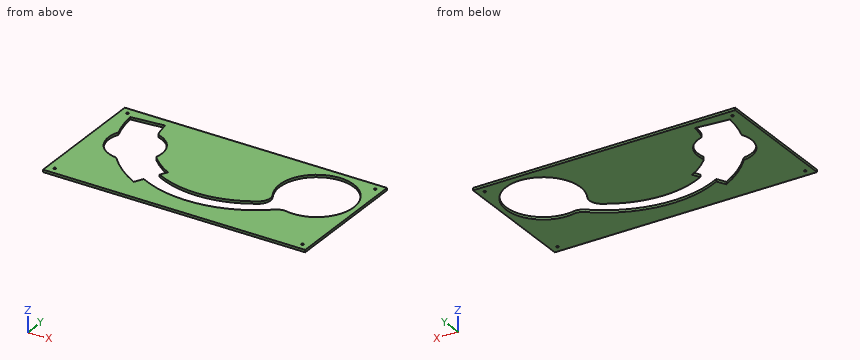
from build123d import *

# Parameters (mm, degrees)
F0_W     = 550
F0_H     = 270
F1_DEPTH = 5
F3_DEPTH = 25
F4_R     = 25
F2_R     = 2.5
F5_DEPTH = 25
F6_R     = 5


with BuildPart() as f1:
    # F0 (on Top) → F1 (new body)
    with BuildSketch(Plane.XY):
        with Locations((275, -135)):
            Rectangle(F0_W, F0_H)
    extrude(amount=-F1_DEPTH)

    # F2 (on face) → F3 (cut)
    with BuildSketch(Plane.XY):
        with BuildLine():
            ThreePointArc((445.5878496959, -168.1072144083), (452.1119253863, -169.1179747106), (458.6981361528, -169.5729777234))
            ThreePointArc((458.6981361528, -169.5729777234), (515.1450884683, -147.5010120731), (538.711061865, -91.6612861494))
            ThreePointArc((538.711061865, -91.6612861494), (531.7751165183, -59.5200686387), (512.2017629268, -33.0994511193))
            ThreePointArc((512.2017629268, -33.0994511193), (489.778644371, -105.9735057557), (445.5878496959, -168.1072144083))
        make_face()
        with BuildLine():
            ThreePointArc((434.4818086721, -165.032732216), (439.9779290015, -166.7755154888), (445.5878496959, -168.1072144083))
            ThreePointArc((445.5878496959, -168.1072144083), (489.778644371, -105.9735057557), (512.2017629268, -33.0994511193))
            ThreePointArc((512.2017629268, -33.0994511193), (507.7316897495, -29.4576002162), (503.004614878, -26.1561769822))
            ThreePointArc((503.004614878, -26.1561769822), (480.8108512866, -101.5487247221), (434.4818086721, -165.032732216))
        make_face()
        with BuildLine():
            ThreePointArc((406.011915497, -147.1219833941), (419.2691571527, -157.6314611673), (434.4818086721, -165.032732216))
            ThreePointArc((434.4818086721, -165.032732216), (480.8108512866, -101.5487247221), (503.004614878, -26.1561769822))
            ThreePointArc((503.004614878, -26.1561769822), (487.87511248, -18.5863859301), (471.4686275556, -14.459543092))
            ThreePointArc((471.4686275556, -14.459543092), (451.6655237624, -87.1681863628), (406.011915497, -147.1219833941))
        make_face()
        with BuildLine():
            ThreePointArc((396.3969974723, -135.5978207964), (400.9264158373, -141.5918788666), (406.011915497, -147.1219833941))
            ThreePointArc((406.011915497, -147.1219833941), (451.6655237624, -87.1681863628), (471.4686275556, -14.459543092))
            ThreePointArc((471.4686275556, -14.459543092), (463.9857274878, -13.7882983897), (456.4729635167, -13.8406471114))
            ThreePointArc((456.4729635167, -13.8406471114), (438.2138341358, -80.5310148123), (396.3969974723, -135.5978207964))
        make_face()
        with BuildLine():
            ThreePointArc((395.2793152892, -133.9137271289), (395.8326968589, -134.7593972826), (396.3969974723, -135.5978207964))
            ThreePointArc((396.3969974723, -135.5978207964), (438.2138341358, -80.5310148123), (456.4729635167, -13.8406471114))
            ThreePointArc((456.4729635167, -13.8406471114), (391.3304963156, -56.2714595868), (395.2793152892, -133.9137271289))
        make_face()
        with BuildLine():
            ThreePointArc((26.1547087534, -24.0004380043), (30.8880481953, -53.9384370008), (39.2095922874, -83.0835942334))
            ThreePointArc((39.2095922874, -83.0835942334), (42.4819606163, -77.1205988593), (46.4524007703, -71.5977994519))
            ThreePointArc((46.4524007703, -71.5977994519), (40.2678425285, -47.5506492992), (36.6062109858, -22.9924196081))
            Line((36.6062109858, -22.9924196081), (26.1547087534, -24.0004380043))
        make_face()
        with BuildLine():
            ThreePointArc((36.6062109858, -22.9924196081), (40.2678425285, -47.5506492992), (46.4524007703, -71.5977994519))
            ThreePointArc((46.4524007703, -71.5977994519), (50.2625511055, -67.3805241048), (54.4801240278, -63.5707031676))
            ThreePointArc((54.4801240278, -63.5707031676), (49.5613274278, -42.9843565598), (46.5600226356, -22.0324020879))
            Line((46.5600226356, -22.0324020879), (36.6062109858, -22.9924196081))
        make_face()
        with BuildLine():
            ThreePointArc((46.5600226356, -22.0324020879), (49.5613274278, -42.9843565598), (54.4801240278, -63.5707031676))
            ThreePointArc((54.4801240278, -63.5707031676), (68.7018719367, -55.1253458568), (84.76908962, -51.1976633843))
            ThreePointArc((84.76908962, -51.1976633843), (81.1661428415, -35.1772059589), (78.9099104977, -18.9123451474))
            Line((78.9099104977, -18.9123451474), (46.5600226356, -22.0324020879))
        make_face()
        with BuildLine():
            ThreePointArc((78.9099104977, -18.9123451474), (81.1661428415, -35.1772059589), (84.76908962, -51.1976633843))
            ThreePointArc((84.76908962, -51.1976633843), (92.7043581114, -51.0322504264), (100.5834584289, -51.9891337337))
            ThreePointArc((100.5834584289, -51.9891337337), (96.3763447636, -34.89397928), (93.8406279725, -17.4723188671))
            Line((93.8406279725, -17.4723188671), (78.9099104977, -18.9123451474))
        make_face()
        with BuildLine():
            ThreePointArc((93.8406279725, -17.4723188671), (96.3763447636, -34.89397928), (100.5834584289, -51.9891337337))
            ThreePointArc((100.5834584289, -51.9891337337), (101.702824577, -52.2182469254), (102.8172889589, -52.4701250099))
            ThreePointArc((102.8172889589, -52.4701250099), (98.4454239564, -35.0497029669), (95.8313903025, -17.2803153631))
            Line((95.8313903025, -17.2803153631), (93.8406279725, -17.4723188671))
        make_face()
        with BuildLine():
            ThreePointArc((102.8172889589, -52.4701250099), (119.1726628165, -90.0990620723), (143.6244940218, -123.0466433063))
            ThreePointArc((143.6244940218, -123.0466433063), (145.375436454, -115.11981647), (145.9631920321, -107.023216784))
            ThreePointArc((145.9631920321, -107.023216784), (133.8730301026, -72.2467564476), (102.8172889589, -52.4701250099))
        make_face()
        with BuildLine():
            ThreePointArc((100.5834584289, -51.9891337337), (117.4412479589, -91.100162762), (142.9268949098, -125.2225814773))
            ThreePointArc((142.9268949098, -125.2225814773), (143.2867819227, -124.1381669965), (143.6244940218, -123.0466433063))
            ThreePointArc((143.6244940218, -123.0466433063), (119.1726628165, -90.0990620723), (102.8172889589, -52.4701250099))
            ThreePointArc((102.8172889589, -52.4701250099), (101.702824577, -52.2182469254), (100.5834584289, -51.9891337337))
        make_face()
        with BuildLine():
            ThreePointArc((84.76908962, -51.1976633843), (104.455636527, -98.6084179347), (135.7230627314, -139.3231306894))
            ThreePointArc((135.7230627314, -139.3231306894), (139.8253147464, -132.5284727964), (142.9268949098, -125.2225814773))
            ThreePointArc((142.9268949098, -125.2225814773), (117.4412479589, -91.100162762), (100.5834584289, -51.9891337337))
            ThreePointArc((100.5834584289, -51.9891337337), (92.7043581114, -51.0322504264), (84.76908962, -51.1976633843))
        make_face()
        with BuildLine():
            ThreePointArc((54.4801240278, -63.5707031676), (76.3201450911, -114.8763041421), (109.8887146149, -159.4004812994))
            ThreePointArc((109.8887146149, -159.4004812994), (124.3031821577, -151.2884347545), (135.7230627314, -139.3231306894))
            ThreePointArc((135.7230627314, -139.3231306894), (104.455636527, -98.6084179347), (84.76908962, -51.1976633843))
            ThreePointArc((84.76908962, -51.1976633843), (68.7018719367, -55.1253458568), (54.4801240278, -63.5707031676))
        make_face()
        with BuildLine():
            ThreePointArc((46.4524007703, -71.5977994519), (67.6630708031, -119.8818075906), (98.9269281749, -162.353082441))
            ThreePointArc((98.9269281749, -162.353082441), (104.4827523758, -161.1549696004), (109.8887146149, -159.4004812994))
            ThreePointArc((109.8887146149, -159.4004812994), (76.3201450911, -114.8763041421), (54.4801240278, -63.5707031676))
            ThreePointArc((54.4801240278, -63.5707031676), (50.2625511055, -67.3805241048), (46.4524007703, -71.5977994519))
        make_face()
        with BuildLine():
            ThreePointArc((39.2095922874, -83.0835942334), (58.5731428007, -125.1375862115), (85.359218008, -162.8998889056))
            ThreePointArc((85.359218008, -162.8998889056), (92.159689712, -163.0387878421), (98.9269281749, -162.353082441))
            ThreePointArc((98.9269281749, -162.353082441), (67.6630708031, -119.8818075906), (46.4524007703, -71.5977994519))
            ThreePointArc((46.4524007703, -71.5977994519), (42.4819606163, -77.1205988593), (39.2095922874, -83.0835942334))
        make_face()
        with BuildLine():
            ThreePointArc((39.2095922874, -83.0835942334), (41.3696850637, -135.0845918815), (85.359218008, -162.8998889056))
            ThreePointArc((85.359218008, -162.8998889056), (58.5731428007, -125.1375862115), (39.2095922874, -83.0835942334))
        make_face()
        with BuildLine():
            ThreePointArc((142.9268949098, -125.2225814773), (165.4491613095, -145.3362093293), (190.9870540226, -161.4491403142))
            Line((190.9870540226, -161.4491403142), (191.9102732092, -159.6749739371))
            ThreePointArc((191.9102732092, -159.6749739371), (166.2146946142, -143.4076613439), (143.6244940218, -123.0466433063))
            ThreePointArc((143.6244940218, -123.0466433063), (143.2867819227, -124.1381669965), (142.9268949098, -125.2225814773))
        make_face()
        with BuildLine():
            ThreePointArc((135.7230627314, -139.3231306894), (158.5376207067, -158.8883702772), (184.0629101234, -174.7553881423))
            Line((184.0629101234, -174.7553881423), (190.9870540226, -161.4491403142))
            ThreePointArc((190.9870540226, -161.4491403142), (165.4491613095, -145.3362093293), (142.9268949098, -125.2225814773))
            ThreePointArc((142.9268949098, -125.2225814773), (139.8253147464, -132.5284727964), (135.7230627314, -139.3231306894))
        make_face()
        with BuildLine():
            ThreePointArc((109.8887146149, -159.4004812994), (137.6857628157, -183.8886898819), (169.0605983417, -203.5855917699))
            Line((169.0605983417, -203.5855917699), (184.0629101234, -174.7553881423))
            ThreePointArc((184.0629101234, -174.7553881423), (158.5376207067, -158.8883702772), (135.7230627314, -139.3231306894))
            ThreePointArc((135.7230627314, -139.3231306894), (124.3031821577, -151.2884347545), (109.8887146149, -159.4004812994))
        make_face()
        with BuildLine():
            ThreePointArc((98.9269281749, -162.353082441), (129.5126452175, -190.2463655327), (164.4445024089, -212.4564236553))
            Line((164.4445024089, -212.4564236553), (169.0605983417, -203.5855917699))
            ThreePointArc((169.0605983417, -203.5855917699), (137.6857628157, -183.8886898819), (109.8887146149, -159.4004812994))
            ThreePointArc((109.8887146149, -159.4004812994), (104.4827523758, -161.1549696004), (98.9269281749, -162.353082441))
        make_face()
        with BuildLine():
            ThreePointArc((85.359218008, -162.8998889056), (119.6639725539, -195.884452107), (159.5976016794, -221.7707971349))
            Line((159.5976016794, -221.7707971349), (164.4445024089, -212.4564236553))
            ThreePointArc((164.4445024089, -212.4564236553), (129.5126452175, -190.2463655327), (98.9269281749, -162.353082441))
            ThreePointArc((98.9269281749, -162.353082441), (92.159689712, -163.0387878421), (85.359218008, -162.8998889056))
        make_face()
        with BuildLine():
            Line((184.0629101234, -174.7553881423), (169.0605983417, -203.5855917699))
            ThreePointArc((169.0605983417, -203.5855917699), (307.9890600374, -227.1166482622), (434.4818086721, -165.032732216))
            ThreePointArc((434.4818086721, -165.032732216), (419.2691571527, -157.6314611673), (406.011915497, -147.1219833941))
            ThreePointArc((406.011915497, -147.1219833941), (299.3392517679, -195.4906668447), (184.0629101234, -174.7553881423))
        make_face()
    extrude(amount=-F3_DEPTH, mode=Mode.SUBTRACT)

    # F4
    f4_edges = [f1.edges().sort_by_distance(p)[0] for p in [
        (406.011915, -147.121983, -2.5),
        (434.481809, -165.032732, -2.5),
    ]]
    fillet(f4_edges, radius=F4_R)

    # F2 (on face) → F5 (cut)
    with BuildSketch(Plane.XY):
        with Locations((15, -15)):
            Circle(F2_R)
        with BuildLine():
            ThreePointArc((17.5, -255), (13.232233047, -253.232233047), (15, -257.5))
            ThreePointArc((15, -257.5), (16.767766953, -256.767766953), (17.5, -255))
        make_face()
        with Locations((535, -255)):
            Circle(F2_R)
        with BuildLine():
            ThreePointArc((537.5, -15), (536.767766953, -13.232233047), (535, -12.5))
            ThreePointArc((535, -12.5), (533.232233047, -16.767766953), (537.5, -15))
        make_face()
    extrude(amount=-F5_DEPTH, mode=Mode.SUBTRACT)

    # F6
    f6_edges = [f1.edges().sort_by_distance(p)[0] for p in [
        (102.817289, -52.470125, -2.5),
        (143.624494, -123.046643, -2.5),
        (39.209592, -83.083594, -2.5),
        (85.359218, -162.899889, -2.5),
    ]]
    fillet(f6_edges, radius=F6_R)


solid = f1.part
For this review, take the finished solid that the model builds, in its own axes (mm). Give positions to 0.01 mm unless a question says otherwise; leave off trailing zeros. Loops run counter-clockwise (first coordinate to the right, second up) from the corner with the lowest first, then second, coordinate; pieces in that order, holes last. Notation, with made-up numbers: (31, -15.75) - (69, -15.75) arc R16 cw to (69, -11.75) - close; hole circle Ø9 at (69.5, -3). An arc over 180 degrees is marked (long way). Write each question's results on one line, items separated by ' | '.
(1) Take a section at A-A (y = -184). Give the boundary of the cut face in (x, z), then the cut area to 3 significant figures.
Conclusion:
outline: (0, -5) - (105.75, -5) - (105.75, 0) - (0, 0) - close; (204.62, -5) - (345.38, -5) - (345.38, 0) - (204.62, 0) - close; (412.17, -5) - (550, -5) - (550, 0) - (412.17, 0) - close | area: 1,920 mm^2
(2) Take a section at B-B (x = 255). Give the boundary of the cut face in (y, z).
Conclusion:
outline: (-270, -5) - (-228.63, -5) - (-228.63, 0) - (-270, 0) - close; (-195.98, -5) - (0, -5) - (0, 0) - (-195.98, 0) - close
(3) For pin 1 Ø6.5 at (x, y) = (535, -255) entering from -Z, flat-tipped, find the tip position at first contact; note if it passes through.
Conclusion:
pin 1: z = -5
(4) For line 1 along Y through (x, z) = (15, -2.75); line 2 along X through (y, z) = (-132.5, -2.3) (3 decimals); line 3 along X through (y, z) = (-152, -0.5), list the stretches that pass through material, from the lowest coordinate up.
Conclusion:
line 1: -270 to -257.5, -252.5 to -17.5, -12.5 to 0 | line 2: 0 to 39.964, 153.165 to 394.179, 527.155 to 550 | line 3: 0 to 56.44, 178.58 to 394.42, 510.11 to 550
(5) Take a section at C-C (z = -3.1). State how many separate pieces and enclosed holes the cut face has, then the cut area to 3 significant figures.
Conclusion:
separate pieces: 1 | enclosed holes: 5 | area: 103,000 mm^2
